Could you check a few things on this model? Use its own coordinates, in mm. A direction names the side the tool comes from. Round coordinates to 2 decimals unless told otherwise and drop trailing zeros. Loops run counter-clockwise (first coordinate to the right, second up) from the corner with the lowest first, then second, coordinate; pieces in that order, holes last. Notation, with made-up numbers: (89, 21) -> (147, 21) arc R21 cw to (147, 33) -> close; hole circle Ø7 at (-33, -1.5). An arc over 180 degrees is marked (long way). Write each question's results on one line, items separated by ' | '. Start each with the question number.
1) Imagine slicing it at A-A, the plane x = 0.5. List the corners of the cut face in (y, z) for me.
2) For P1, Ø4, axis at x = 1, y = -4, coming from the -Z side; P2, Ø3.5, axis at y = -23, z = 0.5, coming from the -X side (3 decimals); P3, Ø1.5, axis at x = 0, y = -15.5, coming from the -Z side, each with a flat end and sliding along its axis, tell me the tip position at first contact or that it passes through.
3) Imagine slicing it at B-B, the plane y = 0.5. List the corners of the cut face in (x, z) for me.
4) Imagine slicing it at C-C, the plane y = -30.5. List the corners of the cut face in (x, z) for me (1 decimal).
5) Which directions (+Z, -Z, +X, -X, +Y, -Y) give clear straight access to the entire face, cutting with the end or side of a thin tool? Please do faces 5 (the flat face through (-1, -2, 0.5)), 6 (the flat face through (-0.925, -24, 1)), 7 (the flat face through (0, -15, 2.049)).
6) If I drill on probe 1 along Y at (x, z) = (0.5, 2.25); probe 2 along Z at (x, y) = (2, -1); probe 3 along X at (y, z) = (-27, 0.75) (3 decimals), over which ranges is the centre line in solid material (lowest first)?
7) We'd pull the mould along Y, two halves only. Please class faces 1 (the cylindrical face through (2.67, -4.7, 1.41)), 2 (the flat face through (0, -24.728, 0)), 3 (the flat face through (0, -24.728, 3)), 4 (the flat face through (0.925, -24, 1)): pulls with the +Y half, pulls with the -Y half, needs draft (parallel to the pull), parting line crosses it, or undercut.
from build123d import *

# Parameters (mm, degrees)
SKETCH_1_R               = 3.532
SKETCH_1_R_2             = 2.165
EXTRUDE_1_DEPTH          = 2.849
EXTRUDE_START            = -2.849
EXTRUDE_3_DEPTH          = 2.849
EXTRUDE_4_DEPTH          = 2.849
SKETCH_5_W               = 4
SKETCH_5_H               = 8.802
EXTRUDE_5_DEPTH          = 2.849
EXTRUDE_6_DEPTH          = 2
EXTRUDE_6_DEPTH_BACK     = 2
SKETCH_11_R              = 2.165
SKETCH_12_W              = 1.376249561
SKETCH_12_H              = 19.360404774
SKETCH_12_W_2            = 1.095086679
CUT_EXTRUDE_1_DEPTH      = 24
CUT_EXTRUDE_2_DEPTH      = 24
CUT_EXTRUDE_2_DEPTH_BACK = 24
SKETCH_14_W              = 1.935032997
SKETCH_14_H              = 19.90949692
SKETCH_14_W_2            = 1.968594382
SKETCH_15_W              = 2.629097519
SKETCH_15_H              = 19.073490401
SKETCH_15_W_2            = 3.221303736
CUT_EXTRUDE_3_DEPTH      = 24
SKETCH_16_W              = 0.5
SKETCH_16_H              = 9.595959473
CUT_EXTRUDE_4_DEPTH      = 24
CUT_EXTRUDE_5_DEPTH      = 24
CUT_EXTRUDE_5_DEPTH_BACK = 24
SKETCH_17_W              = 1.075
SKETCH_17_H              = 30.344064149
SKETCH_19_R              = 2.165
EXTRUDE_7_DEPTH          = 1.849
SKETCH_21_R              = 2.165
EXTRUDE_9_DEPTH          = 1.85


with BuildPart() as part:
    # 草图1 → 凸台-拉伸1 (new body)
    with BuildSketch(Plane.XY):
        Circle(SKETCH_1_R)
        Circle(SKETCH_1_R_2, mode=Mode.SUBTRACT)
    extrude(amount=EXTRUDE_1_DEPTH)

    # 草图3 → 凸台-拉伸3 (add)
    with BuildSketch(Plane.XY.offset(2.849).offset(EXTRUDE_START)):
        with BuildLine():
            Line((-3.323475253, -1.195632151), (-2.916, -3.532))
            ThreePointArc((-2.916, -3.532), (0, -6.448), (2.916, -3.532))
            Line((2.916, -3.532), (3.323475253, -1.195632151))
            ThreePointArc((3.323475253, -1.195632151), (3.042882681, -1.79328999), (2.655959655, -2.328283126))
            ThreePointArc((2.655959655, -2.328283126), (-0.657357457, -3.470288918), (-3.323475253, -1.195632151))
        make_face()
    extrude(amount=EXTRUDE_3_DEPTH)

    # 草图4 → 凸台-拉伸4 (add)
    with BuildSketch(Plane.XY.offset(2.849).offset(EXTRUDE_START)):
        with BuildLine():
            ThreePointArc((2, -5.654040527), (1.075914918, -6.242251481), (0, -6.448))
            Line((0, -6.448), (2, -6.448))
            Line((2, -6.448), (2, -5.654040527))
        make_face()
        with BuildLine():
            Line((0, -6.448), (-2, -6.448))
            Line((-2, -6.448), (-2, -5.654040527))
            ThreePointArc((-2, -5.654040527), (-1.075914918, -6.242251481), (0, -6.448))
        make_face()
    extrude(amount=EXTRUDE_4_DEPTH)

    # 草图5 → 凸台-拉伸5 (add)
    with BuildSketch(Plane.XY.offset(2.849)):
        with Locations((0, -10.849)):
            Rectangle(SKETCH_5_W, SKETCH_5_H)
    extrude(amount=-EXTRUDE_5_DEPTH)

    # 草图11 → 凸台-拉伸6 (add, two sides: drawn at the far end of the back side and taken through both)
    with BuildSketch(Plane.ZY.offset(-EXTRUDE_6_DEPTH_BACK)):
        with BuildLine():
            Line((4.747975253, -29.304367849), (4.3405, -26.968))
            ThreePointArc((4.3405, -26.968), (4.101723935, -25.812349534), (3.4245, -24.845959473))
            Line((3.4245, -24.845959473), (3.4245, -15.25))
            Line((3.4245, -15.25), (-0.5755, -15.25))
            Line((-0.5755, -15.25), (-0.5755, -24.845959473))
            ThreePointArc((-0.5755, -24.845959473), (-1.252723935, -25.812349534), (-1.4915, -26.968))
            Line((-1.4915, -26.968), (-1.898975253, -29.304367849))
            ThreePointArc((-1.898975253, -29.304367849), (1.4245, -34.032), (4.747975253, -29.304367849))
        make_face()
        with Locations((1.4245, -30.5)):
            Circle(SKETCH_11_R, mode=Mode.SUBTRACT)
    extrude(amount=EXTRUDE_6_DEPTH + EXTRUDE_6_DEPTH_BACK)

    # 草图12 → 切除-拉伸1 (cut)
    with BuildSketch(Plane.ZY.offset(12)):
        with Locations((-0.188124781, -5.556058724)):
            Rectangle(SKETCH_12_W, SKETCH_12_H)
        with Locations((2.896543339, -5.556058724)):
            Rectangle(SKETCH_12_W_2, SKETCH_12_H)
    extrude(amount=-CUT_EXTRUDE_1_DEPTH, mode=Mode.SUBTRACT)

    # 草图14 → 切除-拉伸2 (cut, two sides: drawn at the far end of the back side and taken through both)
    with BuildSketch(Plane.XY.offset(3.4245).offset(-CUT_EXTRUDE_2_DEPTH_BACK)):
        with Locations((-2.467516499, -25.20474846)):
            Rectangle(SKETCH_14_W, SKETCH_14_H)
        with Locations((2.484297191, -25.20474846)):
            Rectangle(SKETCH_14_W_2, SKETCH_14_H)
    extrude(amount=CUT_EXTRUDE_2_DEPTH + CUT_EXTRUDE_2_DEPTH_BACK, mode=Mode.SUBTRACT)

    # 草图15 → 切除-拉伸3 (cut)
    with BuildSketch(Plane.ZY.offset(12)):
        with Locations((-0.51454876, -15.190785727)):
            Rectangle(SKETCH_15_W, SKETCH_15_H)
        with Locations((3.659651868, -15.190785727)):
            Rectangle(SKETCH_15_W_2, SKETCH_15_H)
    extrude(amount=-CUT_EXTRUDE_3_DEPTH, mode=Mode.SUBTRACT)

    # 草图16 → 切除-拉伸4 (cut)
    with BuildSketch(Plane(origin=(0, 0, 0.8), x_dir=(-1, 0, 0), z_dir=(0, 0, -1))):
        with Locations((-1.75, -10.452020264)):
            Rectangle(SKETCH_16_W, SKETCH_16_H)
        with Locations((1.75, -10.452020264)):
            Rectangle(SKETCH_16_W, SKETCH_16_H)
    extrude(amount=-CUT_EXTRUDE_4_DEPTH, mode=Mode.SUBTRACT)

    # 草图17 → 切除-拉伸5 (cut, two sides: drawn at the far end of the back side and taken through both)
    with BuildSketch(Plane.XY.offset(2.049).offset(-CUT_EXTRUDE_5_DEPTH_BACK)):
        with Locations((-1.4625, -20.826072602)):
            Rectangle(SKETCH_17_W, SKETCH_17_H)
        with Locations((1.4625, -20.826072602)):
            Rectangle(SKETCH_17_W, SKETCH_17_H)
    extrude(amount=CUT_EXTRUDE_5_DEPTH + CUT_EXTRUDE_5_DEPTH_BACK, mode=Mode.SUBTRACT)

    # 草图19 → 凸台-拉伸7 (add)
    with BuildSketch(Plane(origin=(0, 0, 0.5), x_dir=(-1, 0, 0), z_dir=(0, 0, -1))):
        Circle(SKETCH_19_R)
    extrude(amount=-EXTRUDE_7_DEPTH)

    # 草图18 → 切除-旋转3 (revolve, cut)
    with BuildSketch(Plane(origin=(0, 0, 1.4245), x_dir=(-1, 0, 0), z_dir=(0, 0, -1))):
        with BuildLine():
            Line((0, 2.165), (0, -2.165))
            ThreePointArc((0, -2.165), (-2.165, 0), (0, 2.165))
        make_face()
    revolve(axis=Axis((0, 2.165, 1.4245), (0, -1, 0)), mode=Mode.SUBTRACT)

    # 草图21 → 凸台-拉伸9 (add)
    with BuildSketch(Plane(origin=(0.925, 0, 0), x_dir=(0, 0, -1), z_dir=(1, 0, 0))):
        with Locations((-1.4245, -30.5)):
            Circle(SKETCH_21_R)
    extrude(amount=-EXTRUDE_9_DEPTH)

    # 草图22 → 切除-旋转4 (revolve, cut)
    with BuildSketch(Plane.ZY):
        with BuildLine():
            Line((1.4245, -28.5), (1.4245, -32.5))
            ThreePointArc((1.4245, -32.5), (-0.5755, -30.5), (1.4245, -28.5))
        make_face()
    revolve(axis=Axis((0, -28.5, 1.4245), (0, -1, 0)), mode=Mode.SUBTRACT)


solid = part.part
Checked values:
1) outline: (-29.3, -1.9) -> (-26.97, -1.49) arc R2.92 ccw to (-24.85, -0.58) -> (-24.73, -0.58) -> (-24.73, 0.8) -> (-5.65, 0.8) -> (-5.65, 0.5) -> (-1.89, 0.5) arc R2.11 cw to (-1.89, 2.35) -> (-5.65, 2.35) -> (-5.65, 2.05) -> (-24.73, 2.05) -> (-24.73, 3.42) -> (-24.85, 3.42) arc R2.92 ccw to (-26.97, 4.34) -> (-29.3, 4.75) arc R3.53 ccw (long way) to start; (1.89, 0.5) -> (3.5, 0.5) -> (3.5, 2.35) -> (1.89, 2.35) arc R2.11 cw to start; hole circle Ø3.87 at (-30.5, 1.42)
2) P1: z = 0.5 | P2: x = -0.925 | P3: z = 0.8
3) outline: (-3.5, 0.5) -> (-1.89, 0.5) arc R2.11 cw to (-1.89, 2.35) -> (-3.5, 2.35) -> close; (1.89, 0.5) -> (3.5, 0.5) -> (3.5, 2.35) -> (1.89, 2.35) arc R2.11 cw to start
4) outline: (-0.9, -2.1) -> (0.9, -2.1) -> (0.9, -0.3) arc R2 cw to (-0.9, -0.3) -> close; (-0.9, 3.2) arc R2 cw to (0.9, 3.2) -> (0.9, 5) -> (-0.9, 5) -> close
5) face 5: -Z, +X, -X, +Y | face 6: +Z, -Z, -X, -Y | face 7: +Z, +X, -X
6) probe 1: -33.93 to -32.25, -28.75 to -24.73, -5.65 to -1.94, 1.94 to 3.5 | probe 2: 0.5 to 2.35 | probe 3: -0.925 to 0.925
7) face 1: pulls with the -Y half | face 2: undercut | face 3: undercut | face 4: needs draft
